```python
from build123d import *

# Parameters (mm, degrees)
F2_DEPTH = 50
F3_R     = 25
F4_R     = 24.99999


# Not quite as in the source:
# - a fillet or chamfer is up to 0.001 mm smaller than in the source, because OpenCascade refuses the exact size


with BuildPart() as f2:
    # F1 (on face) → F2 (new body)
    with BuildSketch(Plane.XZ):
        Polygon((8, 80), (0, 80), (0, 0), (86, 0), (86, 10), (61, 10), (36, 10), (36, 34), (28, 34), (28, 10), (8, 10), align=None)
    extrude(amount=F2_DEPTH)

    # F3
    f3_edges = [f2.edges().sort_by_distance(p)[0] for p in [
        (86, -50, 5),
    ]]
    fillet(f3_edges, radius=F3_R)

    # F4 (radius 25 in the source; OpenCascade refuses exactly that, so slightly less here)
    f4_edges = [f2.edges().sort_by_distance(p)[0] for p in [
        (86, 0, 5),
    ]]
    fillet(f4_edges, radius=F4_R)


solid = f2.part
```
Verification items for the finished model (mm, model axes). A direction names the side the tool comes from. Give positions to 0.01 mm unless a question says otherwise; leave off trailing zeros. Order: outer loops, then holes, each group sorted by start corner. A loop starts at its lowest first (then second) coordinate and runs counter-clockwise, first axis right, second up. Notation, with made-up numbers: (-16, 83.5) - (6, 83.5) arc R20 ccw to (6, 117.5) - close; hole circle Ø4 at (-26.75, 88.25). An arc over 180 degrees is marked (long way). Answer as CSV lines item,"result". Start each with the question number.
Item 1: Section check B-B, the plane y = -46.5. Record the boundary of the cut face in (x, z).
Item 2: Material ranges on L1, parallel to X at y = -23.5, z = 30.5; L2, parallel to Z at x = 35, y = -6.5; L3, parallel to Z at x = 82.5, y = -25.5, recorded low to high.
Item 3: Section check D-D, the plane y = -5.5. Record the boundary of the cut face in (x, z), plus the area to 3 significant figures.
Item 4: Section check A-A, the plane z = 12. Record the boundary of the cut face in (x, y), plus the area to 3 significant figures.
Item 5: Gauge pin test, flat ends, axial feed: pin 1 (10 mm diameter, centred on x = 40, y = -29.5, fed in from +Z); pin 2 (19 mm diameter, centred on y = -23.5, z = 20, fed in from +X); pin 3 (5 mm diameter, centred on y = -36.5, z = 47, fed in from +X). Record the tip position at first contact, or that the pin passes through.
Item 6: Access from +Z, -Z, +X, -X, +Y, -Y to the whole of each face (thin tool, end or side, straight path). Record for faces 1 (the face through (18, -25, 10)), 2 (the face through (7.8, -50, 22.4)), 3 (the face through (36, -25, 22)).
Item 7: Mould release check, pull along X, two halves, no side actions. Record for faces 4 (the face through (4, -25, 80)), 5 (the face through (78.871, -42.482, 5.07)), 6 (the face through (8, -25, 45)): released by +X, released by -X, zero draft, split by the parting line, or undercut.
Item 8: Section check C-C, the plane x = 15.5. Record the boundary of the cut face in (y, z), plus the area to 3 significant figures.
Filled in:
1,outline,"(0, 0) - (73.76, 0) - (73.76, 10) - (36, 10) - (36, 34) - (28, 34) - (28, 10) - (8, 10) - (8, 80) - (0, 80) - close"
2,L1,"0 to 8, 28 to 36"
2,L2,"0 to 34"
2,L3,"0 to 10"
3,outline,"(0, 0) - (76.64, 0) - (76.64, 10) - (36, 10) - (36, 34) - (28, 34) - (28, 10) - (8, 10) - (8, 80) - (0, 80) - close"
3,area,"1,520 mm^2"
4,outline,"(0, -50) - (8, -50) - (8, 0) - (0, 0) - close; (28, -50) - (36, -50) - (36, 0) - (28, 0) - close"
4,area,"800 mm^2"
5,pin 1,"z = 34"
5,pin 2,"x = 36"
5,pin 3,"x = 8"
6,face 1,"+Z, +Y, -Y"
6,face 2,"+Z, -Z, +X, -X, -Y"
6,face 3,"+Z, +X, +Y, -Y"
7,face 4,"zero draft"
7,face 5,"released by +X"
7,face 6,"undercut"
8,outline,"(-50, 0) - (0, 0) - (0, 10) - (-50, 10) - close"
8,area,"500 mm^2"
